Source: CAD feature listing. Evaluate the final solid. Frame: model axes, mm. A direction names the side the tool comes from. Give positions to 0.01 mm unless a question says otherwise; leave off trailing zeros. Write each loop counter-clockwise with the first axis right and the second up, starting at its lowest first coordinate (ties: lowest second). Pieces come first, ordered by that corner, then holes. Notation, with made-up numbers: (51, 9.25) -> (77, 9.25) arc R17 ccw to (77, 17.25) -> close; hole circle Ø3 at (50.5, 8.25). An arc over 180 degrees is marked (long way). Answer as a JSON object with one key per item and string values. Group by question number.
Item 1: Section query D-D on z = 65. Return the cut outline in (x, y).
Item 2: Section query A-A on z = 28. Return the cut outline in (x, y), plus the area to 3 significant figures.
Item 3: Section query B-B on x = -145.5. Return the cut outline in (y, z).
Item 4: Ray query, probe 1 along Z at (x, y) = (141.5, -78); probe 2 along X at (y, z) = (101.5, 28.5); probe 3 along X at (y, z) = (153.5, 65). Return the intervals inside material, ascending. Write a range as from..to.
Item 5: Access query for faces 1 (the face through (162.51, 1.82, 7.76)), 2 (the face through (-0.55, 159.86, 77.488)), 3 (the face through (163.986, -144.297, 65.63)). Directions: +Z, -Z, +X, -X, +Y, -Y. A direction counts if a zero-diameter tool reaches every point of the face in a straight line with its end or side. Return the directions, or none.
Item 6: First-contact query: pin 1 Ø16 at (x, z) = (0, 65) entering from +Y; pin 2 Ø1.5 at (x, z) = (50.5, 60) entering from +Y. Flat tips, straight axial feed; report the tip coordinate or a pass-through.
Item 7: Section query C-C on x = 0. Return the cut outline in (y, z), plus the area to 3 significant figures.
Item 8: Pull-direction query (X, two-part tool) for faces 4 (the face through (-164.297, -143.986, 65.63)), 5 (the face through (-2, 147.5, 54)), 6 (the face through (170, -2, 64)); classes: pulls with the +X half, pulls with the -X half, needs draft (parallel to the pull), parting line crosses it, or undercut.
from build123d import *

# Parameters (mm, degrees)
SKETCH1_W           = 340
SKETCH1_H           = 300
BOSS_EXTRUDE1_DEPTH = 130
FILLET1_R           = 20
SKETCH2_R           = 12.5
BOSS_EXTRUDE2_DEPTH = 20
SHELL2_T            = -2.5


with BuildPart() as part:
    # Sketch1 → Boss-Extrude1 (new body)
    with BuildSketch(Plane.XY):
        Rectangle(SKETCH1_W, SKETCH1_H)
    extrude(amount=BOSS_EXTRUDE1_DEPTH)

    # Fillet1
    fillet1_edges = [part.edges().sort_by_distance(p)[0] for p in [
        (-170, 0, 130),
        (0, -150, 130),
        (170, 0, 130),
        (0, -150, 0),
        (-170, 0, 0),
        (0, 150, 0),
        (170, 0, 0),
        (170, -150, 65),
        (-170, -150, 65),
        (-170, 150, 65),
        (170, 150, 65),
        (0, 150, 130),
    ]]
    fillet(fillet1_edges, radius=FILLET1_R)

    # Sketch2 → Boss-Extrude2 (add)
    with BuildSketch(Plane(origin=(0, 150, 0), x_dir=(1, 0, 0), z_dir=(0, 1, 0))):
        with Locations(Location((0, -65, 0), (0, 0, 90))):
            Circle(SKETCH2_R)
    extrude(amount=BOSS_EXTRUDE2_DEPTH)

    # Shell2
    shell2_openings = [part.faces().sort_by_distance(p)[0] for p in [
        (0, 170, 65),
    ]]
    offset(amount=SHELL2_T, openings=shell2_openings, kind=Kind.INTERSECTION)


solid = part.part
Worked answers:
{
 "1": {"outline": "(-170, -130) arc R20 ccw to (-150, -150) -> (150, -150) arc R20 ccw to (170, -130) -> (170, 130) arc R20 ccw to (150, 150) -> (12.5, 150) -> (12.5, 170) -> (10, 170) -> (10, 147.5) -> (150, 147.5) arc R17.5 cw to (167.5, 130) -> (167.5, -130) arc R17.5 cw to (150, -147.5) -> (-150, -147.5) arc R17.5 cw to (-167.5, -130) -> (-167.5, 130) arc R17.5 cw to (-150, 147.5) -> (-10, 147.5) -> (-10, 170) -> (-12.5, 170) -> (-12.5, 150) -> (-150, 150) arc R20 ccw to (-170, 130) -> close"},
 "2": {"outline": "(-170, -130) arc R20 ccw to (-150, -150) -> (150, -150) arc R20 ccw to (170, -130) -> (170, 130) arc R20 ccw to (150, 150) -> (-150, 150) arc R20 ccw to (-170, 130) -> close; hole (-167.5, -130) arc R17.5 ccw to (-150, -147.5) -> (150, -147.5) arc R17.5 ccw to (167.5, -130) -> (167.5, 130) arc R17.5 ccw to (150, 147.5) -> (-150, 147.5) arc R17.5 ccw to (-167.5, 130) -> close", "area": "3,090 mm^2"},
 "3": {"outline": "(-150, 20) arc R20 ccw to (-130, 0) -> (130, 0) arc R20 ccw to (150, 20) -> (150, 110) arc R20 ccw to (130, 130) -> (-130, 130) arc R20 ccw to (-150, 110) -> close; hole (-147.5, 20) arc R17.5 ccw to (-130, 2.5) -> (130, 2.5) arc R17.5 ccw to (147.5, 20) -> (147.5, 110) arc R17.5 ccw to (130, 127.5) -> (-130, 127.5) arc R17.5 ccw to (-147.5, 110) -> close"},
 "4": {"probe 1": "0..2.5, 127.5..130", "probe 2": "-170..-167.5, 167.5..170", "probe 3": "-12.5..-10, 10..12.5"},
 "5": {"face 1": "none", "face 2": "+Y", "face 3": "+Z, -Z, +X, -Y"},
 "6": {"pin 1": "y = -147.5", "pin 2": "y = 150"},
 "7": {"outline": "(-150, 20) arc R20 ccw to (-130, 0) -> (130, 0) arc R20 ccw to (150, 20) -> (150, 52.5) -> (170, 52.5) -> (170, 55) -> (147.5, 55) -> (147.5, 20) arc R17.5 cw to (130, 2.5) -> (-130, 2.5) arc R17.5 cw to (-147.5, 20) -> (-147.5, 110) arc R17.5 cw to (-130, 127.5) -> (130, 127.5) arc R17.5 cw to (147.5, 110) -> (147.5, 75) -> (170, 75) -> (170, 77.5) -> (150, 77.5) -> (150, 110) arc R20 ccw to (130, 130) -> (-130, 130) arc R20 ccw to (-150, 110) -> close", "area": "2,090 mm^2"},
 "8": {"face 4": "pulls with the -X half", "face 5": "undercut", "face 6": "pulls with the +X half"}
}
